The figure shows three views and two pictorial views of one solid part (mm, origin at its lowest corner). Answer the questions. A direction names the side the tool comes from. Coordinates: 2 decimals unless noted, no trailing zeros. Write each loop counter-clockwise with the first axis right and the second up, starting at its lowest first coordinate (ties: lowest second). Pieces come first, ordered by that corner, then holes. Notation, with made-up numbers: (30.5, -24) - (44.5, -24) arc R18 cw to (44.5, -1) - close; hole circle Ø7 at (49, 69). An arc over 180 degrees is marked (long way). Use a Markdown table: item, result. Add a question column.
(1) The part is cut by section B-B, the plane x = 38. Give the vertices of the cut face in (y, z).
(2) The part is cut by section D-D, the plane y = 5. Give the vertices of the cut face in (x, z), then the cut area to 3 significant figures.
(3) The part is cut by section C-C, the plane z = 25. Give the vertices of the cut face in (x, y).
(4) The part is cut by section A-A, the plane y = 52. Give the vertices of the cut face in (x, z), then the cut area to 3 significant figures.
(5) For a pull along X with two mould halves and no side action, classify the marked faces 1, 2 and 3 as released by +X, released by -X, zero draft, split by the parting line, or undercut.
(6) A tool of negligible diameter and unlimited length cuts with its end or side. For the marked faces 4 and 5, from which of +Z, -Z, +X, -X, +Y, -Y can it reach the whole face along a straight path? Write none if from no direction.
(7) Find the intervals of material crossed by line 1 (Y direction, x = 36.5, z = 51.5); line 2 (Z direction, x = 81, y = 46); line 3 (X direction, y = 57, z = 52.5) (3 decimals), in increasing order. Write a range as from..to.
(8) Given pin 1 Ø22.5 at (x, z) = (29.5, 48) entering from -Y; pin 2 Ø2 at (x, y) = (68.5, 25.5) entering from +Z; pin 3 Ø10 at (y, z) = (43.5, 39) entering from -X; pin 4 Ø1 at (x, y) = (59, 21.5) entering from +Z, each flat-ended and moving along its own axis, determine where each tip first touches the part or whether it passes through.
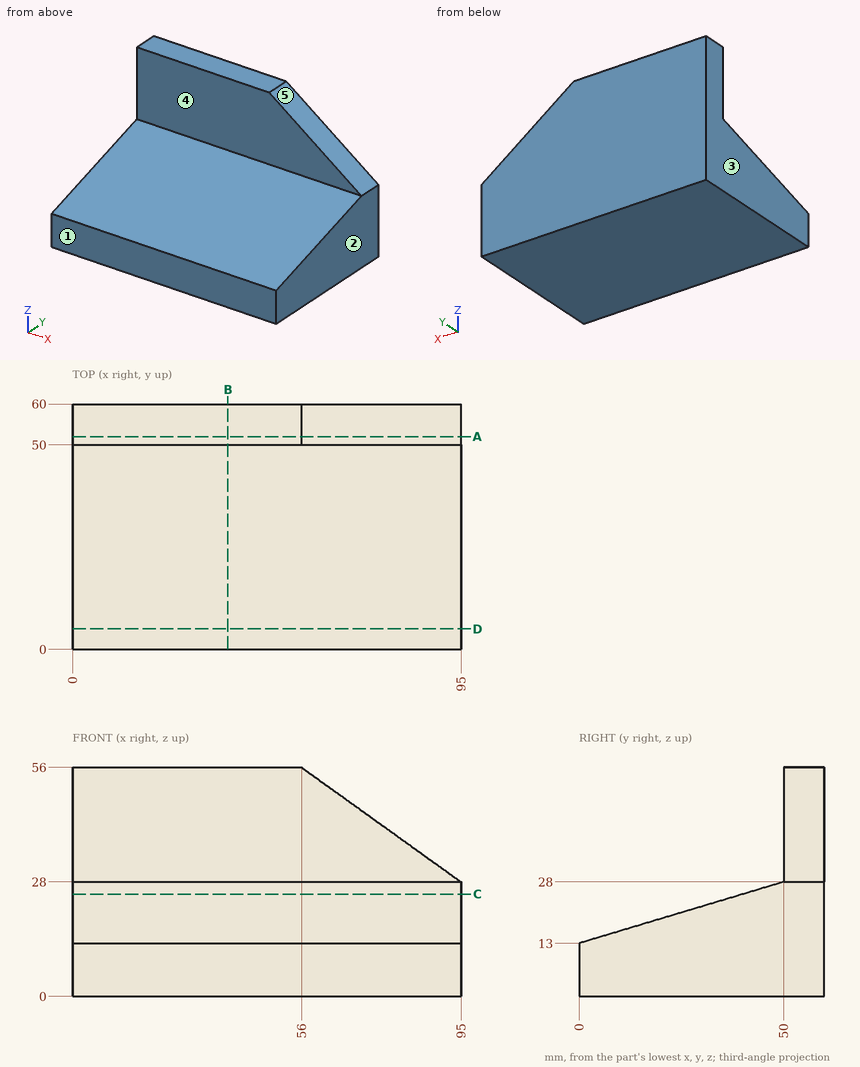
Model answer:
| question | item | result |
|---|---|---|
| 1 | outline | (0, 0) - (60, 0) - (60, 56) - (50, 56) - (50, 28) - (0, 13) - close |
| 2 | outline | (0, 0) - (95, 0) - (95, 14.5) - (0, 14.5) - close |
| 2 | area | 1,380 mm^2 |
| 3 | outline | (0, 40) - (95, 40) - (95, 60) - (0, 60) - close |
| 4 | outline | (0, 0) - (95, 0) - (95, 28) - (56, 56) - (0, 56) - close |
| 4 | area | 4,770 mm^2 |
| 5 | face 1 | zero draft |
| 5 | face 2 | released by +X |
| 5 | face 3 | released by -X |
| 6 | face 4 | +Z, +X, -X, -Y |
| 6 | face 5 | +Z, +X, +Y, -Y |
| 7 | line 1 | 50..60 |
| 7 | line 2 | 0..26.8 |
| 7 | line 3 | 0..60.875 |
| 8 | pin 1 | y = 50 |
| 8 | pin 2 | z = 20.95 |
| 8 | pin 3 | through |
| 8 | pin 4 | z = 19.6 |
